Can you work these out from the drawing? Everything is in mm from the part's minimum corner. Round coordinates to 2 decimals unless told otherwise and drop trailing zeros. Write each loop counter-clockwise with the first axis right and the second up, starting at its lowest first coordinate (ties: lowest second). Pieces come first, ordered by that corner, then holes. Notation, with made-up numbers: (37, -17.75) -> (46, -17.75) arc R11 cw to (46, -9.75) -> close; hole circle Ø9 at (80, -12.5). An arc over 180 degrees is marked (long way). Write item = value, one per line. Start each with the question number.
1) Imagine slicing it at D-D, the plane y = 54.5. Please give me the cut outline in (x, z) (1 decimal).
2) Imagine slicing it at A-A, the plane x = 38.1. State how many separate pieces and enclosed holes the cut face has, then the cut area to 3 significant figures.
3) I'm going to push flat-ended pins straight in: pin 1 (1 mm diameter, centred on x = 54, z = 2, fed in from +Y); pin 2 (1.5 mm diameter, centred on x = 31.5, z = 3, fed in from -Y); pin 3 (1.5 mm diameter, centred on y = 11, z = 2, fed in from -X). Where does each tip first touch, or does it pass through?
4) Imagine slicing it at C-C, the plane z = 1.45. Please give me the cut outline in (x, y) (1 decimal).
5) Imagine slicing it at B-B, the plane y = 38.1. Please give me the cut outline in (x, z) (1 decimal).
6) If I drill on line 1 (Y direction, x = 38, z = 1.8); line 2 (Y direction, x = 17, z = 2.45) (1 decimal); line 3 (X direction, y = 38, z = 1.35), over which ranges is the centre line in solid material (lowest first)?
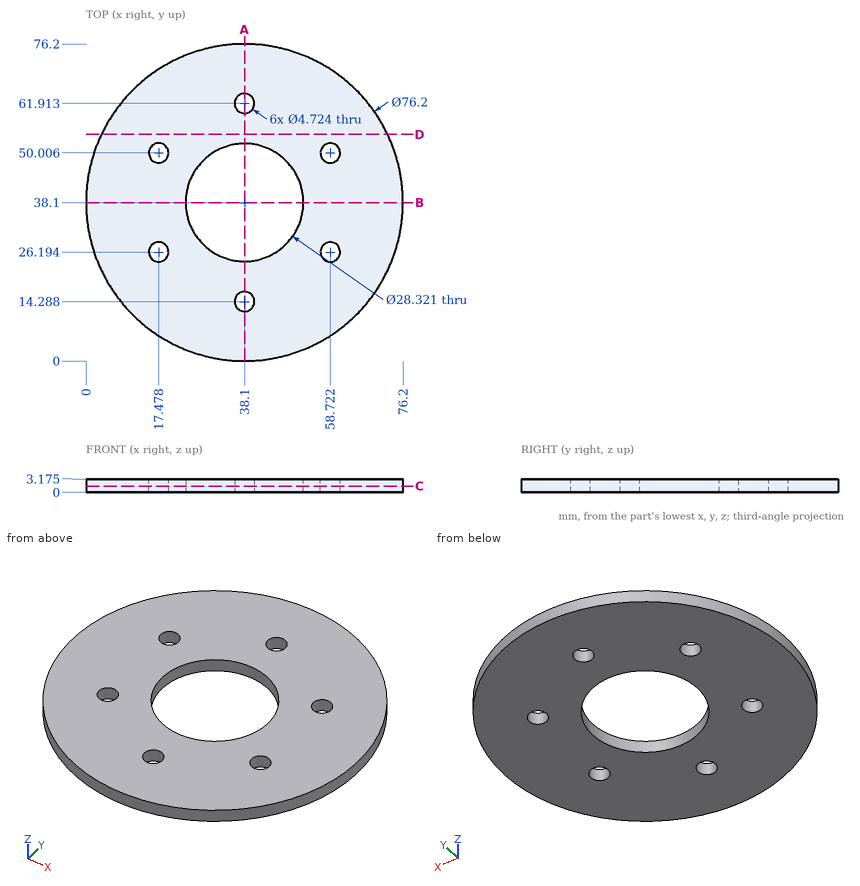
Reported:
q1.outline = (3.7, 0) -> (72.5, 0) -> (72.5, 3.2) -> (3.7, 3.2) -> close
q2.separate_pieces = 4
q2.enclosed_holes = 0
q2.area = 122 mm²
q3.pin_1 = 72.95
q3.pin_2 = 0.45
q3.pin_3 = 10.58
q4.outline = circle Ø76.2 at (38.1, 38.1); hole circle Ø4.7 at (17.5, 26.2); hole circle Ø4.7 at (17.5, 50); hole circle Ø28.3 at (38.1, 38.1); hole circle Ø4.7 at (38.1, 14.3); hole circle Ø4.7 at (38.1, 61.9); hole circle Ø4.7 at (58.7, 26.2); hole circle Ø4.7 at (58.7, 50)
q5.outline = (0, 0) -> (23.9, 0) -> (23.9, 3.2) -> (0, 3.2) -> close; (52.3, 0) -> (76.2, 0) -> (76.2, 3.2) -> (52.3, 3.2) -> close
q6.line_1 = 0 to 11.93, 16.65 to 23.94, 52.26 to 59.55, 64.27 to 76.2
q6.line_2 = 6.4 to 23.9, 28.5 to 47.7, 52.3 to 69.8
q6.line_3 = 0 to 23.94, 52.26 to 76.2
